```python
from build123d import *

# Parameters (mm, degrees)
SKETCH1_W           = 27
SKETCH1_H           = 44
BOSS_EXTRUDE1_DEPTH = 6
CUT_EXTRUDE1_DEPTH  = 27.5
BOSS_EXTRUDE2_DEPTH = 40
BOSS_EXTRUDE3_DEPTH = 40
BOSS_EXTRUDE5_DEPTH = 40
SKETCH6_R           = 2
CUT_EXTRUDE2_DEPTH  = 10
CUT_EXTRUDE3_DEPTH  = 58.697486947
FILLET1_R           = 1
SKETCH5_R           = 2
CUT_EXTRUDE4_DEPTH  = 48.605146781
FILLET2_R           = 3


with BuildPart() as part:
    # Sketch1 → Boss-Extrude1 (new body)
    with BuildSketch(Plane(origin=(0, 0, 0), x_dir=(1, 0, 0), z_dir=(0, 1, 0))):
        Rectangle(SKETCH1_W, SKETCH1_H)
    extrude(amount=BOSS_EXTRUDE1_DEPTH)

    # Sketch2 → Cut-Extrude1 (cut, through all)
    with BuildSketch(Plane(origin=(0, 6, 0), x_dir=(1, 0, 0), z_dir=(0, 1, 0))):
        Polygon((13.5, 22), (-13.5, 6.411542732), (-13.5, 22), align=None)
    extrude(amount=-CUT_EXTRUDE1_DEPTH, mode=Mode.SUBTRACT)

    # Sketch4 → Boss-Extrude2 (add)
    with BuildSketch(Plane(origin=(0, 6, 0), x_dir=(1, 0, 0), z_dir=(0, 1, 0))):
        Polygon((-13.5, 6.411542732), (-13.5, 0.411542732), (13.5, 16), (13.5, 22), align=None)
    extrude(amount=BOSS_EXTRUDE2_DEPTH)

    # Sketch18 → Boss-Extrude3 (add)
    with BuildSketch(Plane(origin=(0, 6, 0), x_dir=(1, 0, 0), z_dir=(0, 1, 0))):
        Polygon((-13.5, -22), (-9.5, -22), (-9.5, 2.720943809), (-13.5, 0.411542732), align=None)
    extrude(amount=BOSS_EXTRUDE3_DEPTH)

    # Sketch19 → Boss-Extrude5 (add)
    with BuildSketch(Plane(origin=(0, 6, 0), x_dir=(1, 0, 0), z_dir=(0, 1, 0))):
        Polygon((13.5, 16), (9.575964778, 13.734457208), (9.575964778, -22), (13.5, -22), align=None)
    extrude(amount=BOSS_EXTRUDE5_DEPTH)

    # Sketch6 → Cut-Extrude2 (cut)
    with BuildSketch(Plane(origin=(-6.151279442, 0, -10.654328524), x_dir=(-0.8660254037844417, 0, 0.4999999999999949), z_dir=(-0.4999999999999949, 0, -0.8660254037844417))):
        with Locations((-6.514428415, 18.5)):
            Circle(SKETCH6_R)
        with Locations((-1.514428415, 31)):
            Circle(SKETCH6_R)
    extrude(amount=-CUT_EXTRUDE2_DEPTH, mode=Mode.SUBTRACT)

    # Sketch20 → Cut-Extrude3 (cut, through all)
    with BuildSketch(Plane.ZY.offset(13.5)):
        Polygon((22, 0), (-2.721542732, 46), (22, 46), align=None)
    extrude(amount=-CUT_EXTRUDE3_DEPTH, mode=Mode.SUBTRACT)

    # Fillet1
    # the kernel refuses this fillet: 1 mm, written as the material it adds along each edge
    with BuildSketch(Plane(origin=(-9.5, 4.556624327, -2.720943809), x_dir=(0.8660254037844415, 0, -0.4999999999999951), z_dir=(0, 1, 0))) as fillet1_piece_1_section:
        with BuildLine():
            CenterArc((FILLET1_R * 0.57735026919, -FILLET1_R), FILLET1_R, 90, 60)
            Line((-FILLET1_R * 0.288675134595, -FILLET1_R * 0.5), (0, 0))
            Line((0, 0), (FILLET1_R * 0.57735026919, 0))
        make_face()
    fillet1_piece_1 = extrude(amount=42.885636914, mode=Mode.PRIVATE)
    fillet1_piece_1 = split(fillet1_piece_1, bisect_by=Plane(origin=(-9.391668289, 14.377701734, 14.273065917), z_dir=(0, -0.47339174882638807, -0.8808520035415109)), keep=Keep.TOP, mode=Mode.PRIVATE)
    fillet1_piece_1 = split(fillet1_piece_1, bisect_by=Plane(origin=(-9.391668289, 46, -2.658398466), z_dir=(0, -1, 0)), keep=Keep.TOP, mode=Mode.PRIVATE)
    add(fillet1_piece_1)
    with BuildSketch(Plane(origin=(9.575964778, 1.669872981, -13.734457208), x_dir=(-0.8660254037844415, 0, 0.4999999999999951), z_dir=(0, 1, 0))) as fillet1_piece_2:
        with BuildLine():
            CenterArc((FILLET1_R * 1.73205080757, FILLET1_R), FILLET1_R, 150, 120)
            Line((FILLET1_R * 0.866025403784, FILLET1_R * 1.5), (0, 0))
            Line((0, 0), (FILLET1_R * 1.73205080757, 0))
        make_face()
    extrude(amount=44.330127019)

    # Sketch5 → Cut-Extrude4 (cut, through all)
    with BuildSketch(Plane(origin=(0, 6, 0), x_dir=(1, 0, 0), z_dir=(0, 1, 0))):
        with Locations(Location((-5.5, -12, 0), (0, 0, 270))):
            Circle(SKETCH5_R)
        with Locations(Location((4.5, -2, 0), (0, 0, 270))):
            Circle(SKETCH5_R)
    extrude(amount=-CUT_EXTRUDE4_DEPTH, mode=Mode.SUBTRACT)

    # Fillet2
    # the kernel refuses this fillet: 3 mm, written as the material it takes off along each edge
    with BuildSketch(Plane(origin=(5.092167423, 46, -2.721542732), x_dir=(0, 0, -1), z_dir=(1, 0, 0))) as fillet2_piece_1:
        with BuildLine():
            CenterArc((FILLET2_R * 0.59783964736, -FILLET2_R), FILLET2_R, 90, 61.74531149)
            Line((-FILLET2_R * 0.283012356181, -FILLET2_R * 0.526608251174), (0, 0))
            Line((0, 0), (FILLET2_R * 0.59783964736, 0))
        make_face()
    extrude(amount=12.891629932, mode=Mode.SUBTRACT)
    with BuildSketch(Plane(origin=(-17.983797355, 46, -2.721542732), x_dir=(0, 0, -1), z_dir=(1, 0, 0))) as fillet2_piece_2:
        with BuildLine():
            CenterArc((FILLET2_R * 0.59783964736, -FILLET2_R), FILLET2_R, 90, 61.74531149)
            Line((-FILLET2_R * 0.283012356181, -FILLET2_R * 0.526608251174), (0, 0))
            Line((0, 0), (FILLET2_R * 0.59783964736, 0))
        make_face()
    extrude(amount=8.484834721, mode=Mode.SUBTRACT)
    with BuildSketch(Plane(origin=(-4.832275393, 46, -2.721542732), x_dir=(0, 0, -1), z_dir=(-1, 0, 0))) as fillet2_piece_3:
        with BuildLine():
            CenterArc((FILLET2_R * 0.59783964736, FILLET2_R), FILLET2_R, 208.25468851, 61.74531149)
            Line((-FILLET2_R * 0.283012356181, FILLET2_R * 0.526608251174), (0, 0))
            Line((0, 0), (FILLET2_R * 0.59783964736, 0))
        make_face()
    extrude(amount=4.666687241, mode=Mode.SUBTRACT)


solid = part.part
```
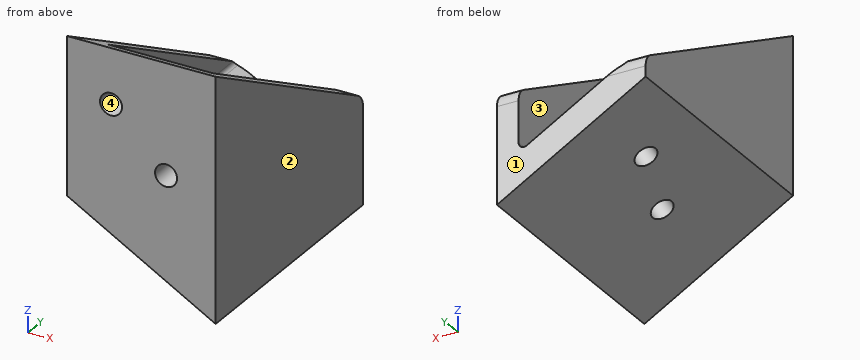
CAD build for the part. Positions are in the model's coordinates, mm. Face numbers are marked on the shaded views. Coordinates: 2 decimals unless noted, no trailing zeros. Order: outer loops, then holes, each group sorted by start corner. A loop starts at its lowest first (then second) coordinate and runs counter-clockwise, first axis right, second up.
(1) Pin check, flat tips, straight feed: pin 1 Ø2 at (x, y) = (-0.5, 5) entering from +Z; pin 2 Ø3 at (x, y) = (-3.5, 5) entering from -Z; pin 3 Ø2 at (x, y) = (-7.5, 19.5) entering from +Z; pin 4 Ø6.5 at (x, z) = (4.5, 2) entering from -Y. Stop position of each tip, or through.
Solution:
pin 1: stops at z = 19.85
pin 2: stops at z = -13.05
pin 3: stops at z = -3.3
pin 4: stops at y = 0
(2) Saw through at D-D, the plane z = 2. Write the cut outline in (x, y), and give its area (3 significant figures).
Solution:
outline: (-13.5, 0) - (2.5, 0) - (2.5, 6) - (-9.5, 6) - (-9.5, 37.21) - (-13.5, 37.21) - close; (6.5, 0) - (13.5, 0) - (13.5, 37.21) - (9.58, 37.21) - (9.58, 6) - (6.5, 6) - close
area: 385 mm2
(3) Mould opens along X. For the marked faces 1, 2, 3 and 4 say: released by +X, released by -X, zero draft, split by the parting line, or undercut.
Solution:
face 1: zero draft
face 2: released by +X
face 3: undercut
face 4: undercut
(4) Saw through at C-C, the plane y = 30. Write the cut outline in (x, z), and give its area (3 significant figures).
Solution:
outline: (-13.5, -6.41) - (-6.34, -10.55) - (-3.74, -6.05) - (-9, -3.01) arc R1 cw to (-9.5, -2.14) - (-9.5, 5.88) - (-13.5, 5.88) - close; (-3.34, -12.28) - (13.5, -22) - (13.5, 5.88) - (9.58, 5.88) - (9.58, -12) arc R1 cw to (8.08, -12.87) - (-0.74, -7.78) - close
area: 256 mm2
(5) Saw through at A-A, the plane z = 11.5. Write the cut outline in (x, y), and give its area (3 significant figures).
Solution:
outline: (-13.5, 0) - (-7.44, 0) - (-7.44, 6) - (-9.5, 6) - (-9.5, 19.54) - (-13.5, 19.54) - close; (-3.56, 0) - (13.5, 0) - (13.5, 19.54) - (9.58, 19.54) - (9.58, 6) - (-3.56, 6) - close
area: 246 mm2
(6) Saw through at B-B, the plane x = 4.5. Write the cut outline in (y, z).
Solution:
outline: (0, -16.8) - (46, -16.8) - (46, -10.8) - (6, -10.8) - (6, 0) - (0, 0) - close; (0, 4) - (6, 4) - (6, 18.78) - (0, 22) - close
(7) Drill centre lines: L1, parallel to Y at x = -2.5, z = -7; L2, parallel to X at y = 3.15, z = 12; L3, parallel to X at y = 3.7, z = 2. Where is each one in solid material? Low to high.
Solution:
L1: y = 0 to 29.01, 32.99 to 46
L2: x = -13.5 to -7.5, -3.5 to 13.5
L3: x = -13.5 to 2.5, 6.5 to 13.5
